```python
from build123d import *

# Parameters (mm, degrees)
BOSS_EXTRUDE1_DEPTH            = 26.8
SKETCH2_W                      = 21.5
SKETCH2_H                      = 43.5
SKETCH2_W_2                    = 43.5
SKETCH2_H_2                    = 21.5
CUT_EXTRUDE1_DEPTH             = 169.899357105
SKETCH3_R                      = 1.15
BOSS_EXTRUDE2_DEPTH            = 26.8
SKETCH3_2_R                    = 1.15
CUT_EXTRUDE2_DEPTH             = 169.899357105
SKETCH4_R                      = 1.15
CUT_EXTRUDE3_DEPTH             = 169.899357105
FILLET2_R                      = 2
CBORE_FOR_M3_SHCS1_D           = 3.4
CBORE_FOR_M3_SHCS1_CBORE_D     = 6.5
CBORE_FOR_M3_SHCS1_CBORE_DEPTH = 3
SKETCH12_W                     = 14
SKETCH12_H                     = 14
CUT_EXTRUDE5_DEPTH             = 10
SKETCH13_W                     = 13
SKETCH13_H                     = 13
CUT_EXTRUDE6_DEPTH             = 168.603677855
SKETCH14_R                     = 3.585
CUT_EXTRUDE7_DEPTH             = 169.899357105


with BuildPart() as part:
    # Sketch1 → Boss-Extrude1 (new body)
    with BuildSketch(Plane.XY):
        Polygon((85.79616933, 12.865007186), (115.79616933, 12.865007186), (115.79616933, 119.999999996), (85.79616933, 119.999999996), (85.79616933, 42.865007186), (5.79616933, 42.865007186), (5.79616933, 119.999999996), (-24.20383067, 119.999999996), (-24.20383067, 12.865007186), (5.79616933, 12.865007186), align=None)
    extrude(amount=BOSS_EXTRUDE1_DEPTH)

    # Sketch2 → Cut-Extrude1 (cut, through all)
    with BuildSketch(Plane.XY.offset(26.8)):
        with Locations((-9.20383067, 61.615007186)):
            Rectangle(SKETCH2_W, SKETCH2_H)
        with Locations((57.04616933, 28.145492547)):
            Rectangle(SKETCH2_W_2, SKETCH2_H_2)
    extrude(amount=-CUT_EXTRUDE1_DEPTH, mode=Mode.SUBTRACT)

    # Sketch3 → Boss-Extrude2 (add, through all)
    with BuildSketch(Plane.XY.offset(26.8)):
        with Locations((-14.20383067, 34.565007186)):
            Circle(SKETCH3_R)
        with Locations((-4.20383067, 34.565007186)):
            Circle(SKETCH3_R)
        with Locations((-14.20383067, 85.665007186)):
            Circle(SKETCH3_R)
        with Locations((-4.20383067, 85.665007186)):
            Circle(SKETCH3_R)
    extrude(amount=-BOSS_EXTRUDE2_DEPTH)

    # Sketch3<2> → Cut-Extrude2 (cut, through all)
    with BuildSketch(Plane.XY.offset(26.8)):
        with Locations((-14.20383067, 34.565007186)):
            Circle(SKETCH3_2_R)
        with Locations((-4.20383067, 34.565007186)):
            Circle(SKETCH3_2_R)
        with Locations((-14.20383067, 85.665007186)):
            Circle(SKETCH3_2_R)
        with Locations(Location((-4.20383067, 85.665007186, 0), (0, 0, 180))):
            Circle(SKETCH3_2_R)
    extrude(amount=-CUT_EXTRUDE2_DEPTH, mode=Mode.SUBTRACT)

    # Sketch4 → Cut-Extrude3 (cut, through all)
    with BuildSketch(Plane.XY.offset(26.8)):
        with Locations((84.09616933, 23.145492547)):
            Circle(SKETCH4_R)
        with Locations(Location((84.09616933, 33.145492547, 0), (0, 0, 180))):
            Circle(SKETCH4_R)
        with Locations((32.99616933, 23.145492547)):
            Circle(SKETCH4_R)
        with Locations(Location((32.99616933, 33.145492547, 0), (0, 0, 180))):
            Circle(SKETCH4_R)
    extrude(amount=-CUT_EXTRUDE3_DEPTH, mode=Mode.SUBTRACT)

    # Fillet2
    fillet2_edges = [part.edges().sort_by_distance(p)[0] for p in [
        (85.79616933, 81.432503591, 0),
        (100.79616933, 119.999999996, 0),
        (115.79616933, 66.432503591, 0),
        (45.79616933, 12.865007186, 0),
        (-24.20383067, 66.432503591, 0),
        (-9.20383067, 119.999999996, 0),
        (5.79616933, 81.432503591, 0),
        (45.79616933, 42.865007186, 0),
    ]]
    fillet(fillet2_edges, radius=FILLET2_R)

    # CBORE for M3 SHCS1 (through all)
    with Locations(Plane(origin=(0, 0, 0), x_dir=(-1, 0, 0), z_dir=(0, 0, -1))):
        with Locations((-25.79616933, 27.865007186), (9.20383067, 109.999999996), (-100.79616933, 109.999999996)):
            CounterBoreHole(CBORE_FOR_M3_SHCS1_D / 2, CBORE_FOR_M3_SHCS1_CBORE_D / 2, CBORE_FOR_M3_SHCS1_CBORE_DEPTH)

    # Sketch12 → Cut-Extrude5 (cut)
    with BuildSketch(Plane(origin=(0, 0, 0), x_dir=(-1, 0, 0), z_dir=(0, 0, -1))):
        with Locations((-100.79616933, 84.999999996)):
            Rectangle(SKETCH12_W, SKETCH12_H)
    extrude(amount=-CUT_EXTRUDE5_DEPTH, mode=Mode.SUBTRACT)

    # Sketch13 → Cut-Extrude6 (cut, through all)
    with BuildSketch(Plane(origin=(0, 0, 10), x_dir=(-1, 0, 0), z_dir=(0, 0, -1))):
        with Locations((-100.79616933, 84.999999996)):
            Rectangle(SKETCH13_W, SKETCH13_H)
    extrude(amount=-CUT_EXTRUDE6_DEPTH, mode=Mode.SUBTRACT)

    # Sketch14 → Cut-Extrude7 (cut, through all)
    with BuildSketch(Plane(origin=(0, 0, 0), x_dir=(-1, 0, 0), z_dir=(0, 0, -1))):
        with Locations((-100.79616933, 64.999999996)):
            Circle(SKETCH14_R)
    extrude(amount=-CUT_EXTRUDE7_DEPTH, mode=Mode.SUBTRACT)


solid = part.part
```
CAD build for the part. Positions are in the model's coordinates, mm. A direction names the side the tool comes from. Round coordinates to 2 decimals unless told otherwise and drop trailing zeros. Loops run counter-clockwise (first coordinate to the right, second up) from the corner with the lowest first, then second, coordinate; pieces in that order, holes last. Notation, with made-up numbers: (-21.75, 47.5) - (0.25, 47.5) arc R27 cw to (0.25, 83.5) - close; hole circle Ø10 at (-18.75, -30.5). An arc over 180 degrees is marked (long way). Return JSON: item names as keys, results as strings. Group by question number.
Q1. Drill centre lines: line 1 along X through (y, z) = (65, 20.5); line 2 along X through (y, z) = (74, 20.5); line 3 along Y through (x, z) = (84, 2.75) (3 decimals). Where is each one in solid material? Low to high. Write a range as [from, to].
Q2. Band-saw the part on C-C on z = 25.25. Give the number of separate pieces and of enclosed holes in the cut face, plus the area to 3 significant figures.
Q3. Band-saw the part on A-A on x = 55.5. Give the cut face in (y, z) (1 decimal), plus the area to 3 significant figures.
Q4. Flat gauge pins, fed straight in: pin 1 Ø1.8 at (x, y) = (-14.2, 34.57) entering from -Z; pin 2 Ø6 at (x, z) = (53, 21) entering from +Y (3 decimals); pin 3 Ø7.5 at (x, y) = (100.8, 110) entering from +Z; pin 4 Ø2 at (x, y) = (100, 109.5) entering from -Z. Where does each tip first touch, or does it go through?
Q5. Tool access for faces 1 (the face through (26.219, 31.087, 1.479)), 2 (the face through (46, 42.865, 14)), 3 (the face through (1.546, 61, 14)), 4 (the face through (-24.204, 67, 14)): list every direction of +Z, -Z, +X, -X, +Y, -Y with a clear straight run to the whole face (end or side of a thin tool).
Q6. Band-saw the part on D-D on y = 110. Give the cut face in (x, z), plus the area to 3 significant figures.
Q7. Two-plate mould, pull along X, no slides. Class faces 5 (the face through (115.796, 66, 14)), 6 (the face through (24.098, 27.94, 15.067)), 7 (the face through (30, 33, 0)), 8 (the face through (107.296, 85, 18)): +X half, -X half, draft (parallel to the pull), parting line (faces both ways), or undercut.
Q8. Band-saw the part on B-B on y = 65. Give the cut face in (x, z), plus the area to 3 significant figures.
Solutions:
{
 "1": {"line 1": "x = [-24.2, -19.95], [1.55, 5.8], [85.8, 97.21], [104.38, 115.8]", "line 2": "x = [-24.2, -19.95], [1.55, 5.8], [85.8, 115.8]", "line 3": "y = [12.865, 22], [24.291, 32], [34.291, 42.865]"},
 "2": {"separate pieces": "1", "enclosed holes": "15", "area": "6,690 mm^2"},
 "3": {"outline": "(12.9, 2) arc R2 ccw to (14.9, 0) - (17.4, 0) - (17.4, 26.8) - (12.9, 26.8) - close; (38.9, 0) - (40.9, 0) arc R2 ccw to (42.9, 2) - (42.9, 26.8) - (38.9, 26.8) - close", "area": "226 mm^2"},
 "4": {"pin 1": "passes through", "pin 2": "stops at y = 42.865", "pin 3": "stops at z = 26.8", "pin 4": "stops at z = 3"},
 "5": {"face 1": "-Z", "face 2": "+Z, -Z, +Y", "face 3": "+Z, -Z", "face 4": "+Z, -Z, -X, +Y, -Y"},
 "6": {"outline": "(-24.2, 2) arc R2 ccw to (-22.2, 0) - (-12.45, 0) - (-12.45, 3) - (-10.9, 3) - (-10.9, 26.8) - (-24.2, 26.8) - close; (-7.5, 3) - (-5.95, 3) - (-5.95, 0) - (3.8, 0) arc R2 ccw to (5.8, 2) - (5.8, 26.8) - (-7.5, 26.8) - close; (85.8, 2) arc R2 ccw to (87.8, 0) - (97.55, 0) - (97.55, 3) - (99.1, 3) - (99.1, 26.8) - (85.8, 26.8) - close; (102.5, 3) - (104.05, 3) - (104.05, 0) - (113.8, 0) arc R2 ccw to (115.8, 2) - (115.8, 26.8) - (102.5, 26.8) - close", "area": "1,400 mm^2"},
 "7": {"face 5": "+X half", "face 6": "undercut", "face 7": "draft", "face 8": "undercut"},
 "8": {"outline": "(-24.2, 2) arc R2 ccw to (-22.2, 0) - (-19.95, 0) - (-19.95, 26.8) - (-24.2, 26.8) - close; (1.55, 0) - (3.8, 0) arc R2 ccw to (5.8, 2) - (5.8, 26.8) - (1.55, 26.8) - close; (85.8, 2) arc R2 ccw to (87.8, 0) - (97.21, 0) - (97.21, 26.8) - (85.8, 26.8) - close; (104.38, 0) - (113.8, 0) arc R2 ccw to (115.8, 2) - (115.8, 26.8) - (104.38, 26.8) - close", "area": "836 mm^2"}
}
